```python
from build123d import *

# Parameters (mm, degrees)
SKETCH1_R           = 6.223
BOSS_EXTRUDE1_DEPTH = 4.7498
SKETCH2_R           = 3.683
BOSS_EXTRUDE2_DEPTH = 7.0104
SKETCH3_R           = 6.223
BOSS_EXTRUDE3_DEPTH = 4.7498
SKETCH4_R           = 2.54
CUT_EXTRUDE1_DEPTH  = 16.51


with BuildPart() as part:
    # Sketch1 → Boss-Extrude1 (new body)
    with BuildSketch(Plane(origin=(0, 0, 0), x_dir=(1, 0, 0), z_dir=(0, 1, 0))):
        Circle(SKETCH1_R)
    extrude(amount=BOSS_EXTRUDE1_DEPTH)

    # Sketch2 → Boss-Extrude2 (add)
    with BuildSketch(Plane(origin=(0, 4.7498, 0), x_dir=(1, 0, 0), z_dir=(0, 1, 0))):
        Circle(SKETCH2_R)
    extrude(amount=BOSS_EXTRUDE2_DEPTH)

    # Sketch3 → Boss-Extrude3 (add)
    with BuildSketch(Plane(origin=(0, 11.7602, 0), x_dir=(1, 0, 0), z_dir=(0, 1, 0))):
        Circle(SKETCH3_R)
    extrude(amount=BOSS_EXTRUDE3_DEPTH)

    # Sketch4 → Cut-Extrude1 (cut)
    with BuildSketch(Plane(origin=(0, 16.51, 0), x_dir=(1, 0, 0), z_dir=(0, 1, 0))):
        Circle(SKETCH4_R)
    extrude(amount=-CUT_EXTRUDE1_DEPTH, mode=Mode.SUBTRACT)

    # Sketch5 → Cut-Revolve1 (revolve, cut)
    with BuildSketch(Plane(origin=(0, 0, 0), x_dir=(0, 0, -1), z_dir=(1, 0, 0))):
        Polygon((0, 16.51), (0, 13.716), (2.54, 13.716), (4.5974, 16.51), align=None)
    revolve(axis=Axis((0, 16.51, 0), (0, -1, 0)), mode=Mode.SUBTRACT)


solid = part.part
```
Geometry: final body of the model. Coordinates: model frame, mm. A direction names the side the tool comes from. Round coordinates to 2 decimals unless told otherwise and drop trailing zeros. Order: outer loops, then holes, each group sorted by start corner. A loop starts at its lowest first (then second) coordinate and runs counter-clockwise, first axis right, second up. Notation, with made-up numbers: (31, 36.25) -> (54, 36.25) arc R31 ccw to (54, 69.25) -> close; hole circle Ø1 at (77, -6). An arc over 180 degrees is marked (long way). Use CSV: the item, a comma, the result in double quotes. Start each with the question number.
1) First-contact query: pin 1 Ø6.5 at (x, z) = (0, 0) entering from +Y; pin 2 Ø1.5 at (x, z) = (1, 3) entering from +Y. Flat tips, straight axial feed; report the tip coordinate or a pass-through.
2) Section C-C (y = 3.75). Return the cut outline in (x, z).
3) Section B-B (x = 0). Return the cut outline in (y, z), and give its area (3 significant figures).
4) Material intervals for line 1 along Z through (x, y) = (0, 6); line 2 along Y through (x, z) = (5, 0.5), sorted ascending. Write a range as from..to.
5) Set-up query: faces 5 (the face through (3, 11.76, 3)), 6 (the face through (0, 0, 3)). Return all of +Z, -Z, +X, -X, +Y, -Y with unobstructed straight access to the full face (end or side cutting, diameter ignored); none if empty.
6) Section D-D (y = 11.25). Return the cut outline in (x, z).
7) Section A-A (z = 0). Return the cut outline in (x, y), and give its area (3 significant figures).
8) Draft query along Z for faces 1 (the face through (3, 4.75, 3)), 2 (the face through (1.699, 8.206, 3.267)), 3 (the face through (2.423, 6.954, -0.763)), 4 (the face through (0.802, 13.891, -2.545)). Return one class per face: +Z half, -Z half, draft (parallel to the pull), parting line (faces both ways), or undercut.
Returned:
1,pin 1,"stops at y = 14.68"
1,pin 2,"stops at y = 15.58"
2,outline,"circle Ø12.45 at (0, 0); hole circle Ø5.08 at (0, 0)"
3,outline,"(0, -6.22) -> (4.75, -6.22) -> (4.75, -3.68) -> (11.76, -3.68) -> (11.76, -6.22) -> (16.51, -6.22) -> (16.51, -4.6) -> (13.72, -2.54) -> (0, -2.54) -> close; (0, 2.54) -> (13.72, 2.54) -> (16.51, 4.6) -> (16.51, 6.22) -> (11.76, 6.22) -> (11.76, 3.68) -> (4.75, 3.68) -> (4.75, 6.22) -> (0, 6.22) -> close"
3,area,"80.3 mm²"
4,line 1,"z = -3.68..-2.54, 2.54..3.68"
4,line 2,"y = 0..4.75, 11.76..16.51"
5,face 5,"none"
5,face 6,"+Z, -Z, +X, -X, -Y"
6,outline,"circle Ø7.37 at (0, 0); hole circle Ø5.08 at (0, 0)"
7,outline,"(-6.22, 0) -> (-2.54, 0) -> (-2.54, 13.72) -> (-4.6, 16.51) -> (-6.22, 16.51) -> (-6.22, 11.76) -> (-3.68, 11.76) -> (-3.68, 4.75) -> (-6.22, 4.75) -> close; (2.54, 0) -> (6.22, 0) -> (6.22, 4.75) -> (3.68, 4.75) -> (3.68, 11.76) -> (6.22, 11.76) -> (6.22, 16.51) -> (4.6, 16.51) -> (2.54, 13.72) -> close"
7,area,"80.3 mm²"
8,face 1,"draft"
8,face 2,"parting line"
8,face 3,"undercut"
8,face 4,"undercut"
